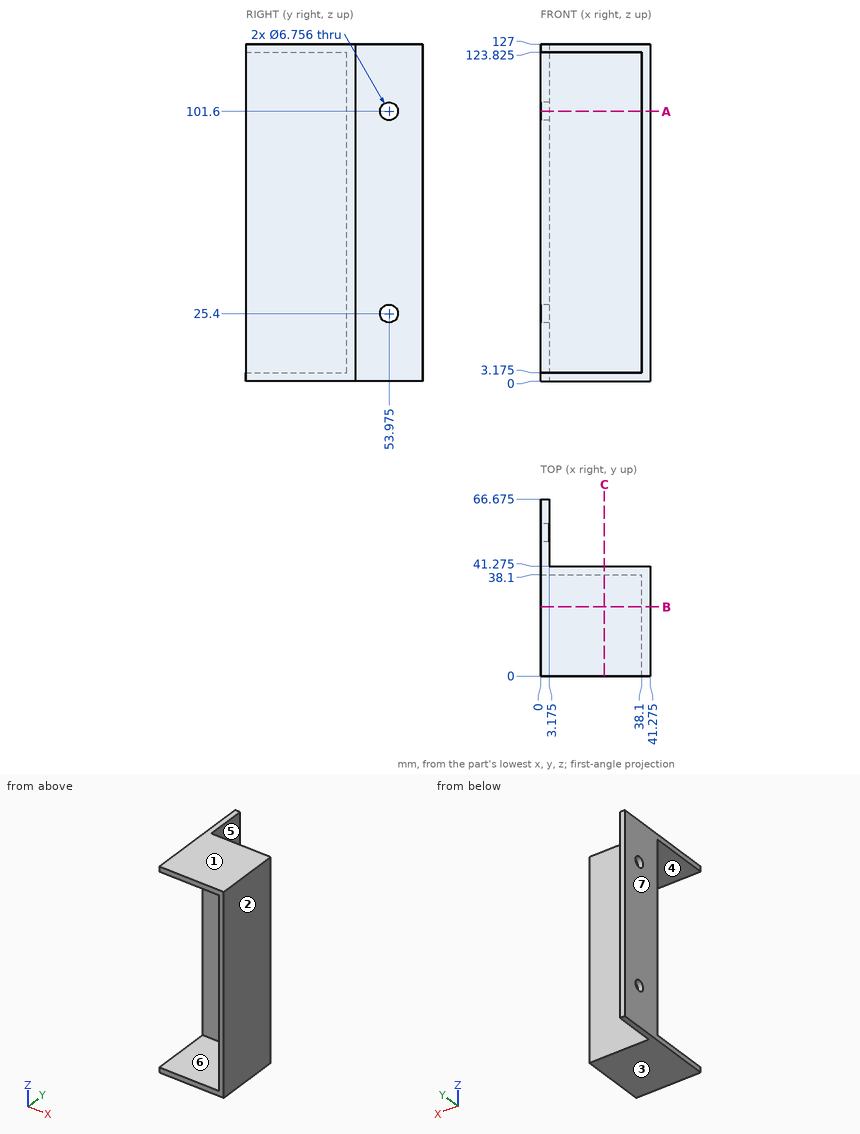
Source: three-view drawing plus pictorial views. Frame: mm from the lowest corner of the part. A direction names the side the tool comes from. Coordinates: 2 decimals unless noted, no trailing zeros. Order: outer loops, then holes, each group sorted by start corner. A loop starts at its lowest first (then second) coordinate and runs counter-clockwise, first axis right, second up.
Item 1: Set-up query: the marked faces 5, 6 and 7. Return all of +Z, -Z, +X, -X, +Y, -Y with unobstructed straight access to the full face (end or side cutting, diameter ignored); none if empty.
Output values:
face 5: +Z, -Z, +X, +Y
face 6: -X, -Y
face 7: +Z, -Z, -X, +Y, -Y
Item 2: Cut plane A-A (z = 101.6). Return loops of the section in (x, y) (1 decimal).
Output values:
outline: (0, 38.1) - (38.1, 38.1) - (38.1, 0) - (41.3, 0) - (41.3, 41.3) - (3.2, 41.3) - (3.2, 50.6) - (0, 50.6) - close; (0, 57.4) - (3.2, 57.4) - (3.2, 66.7) - (0, 66.7) - close
Item 3: Material intervals for line 1 (Y direction, x = 1.4, z = 101.6) (1 decimal); line 2 (Z direction, x = 4, y = 24) (1 decimal); line 3 (Y direction, x = 2, z = 25) (1 decimal), sorted ascending.
Output values:
line 1: y = 38.1 to 50.6, 57.4 to 66.7
line 2: z = 0 to 3.2, 123.8 to 127
line 3: y = 38.1 to 50.6, 57.3 to 66.7
Item 4: Cut plane B-B (y = 26). Return loops of the section in (x, z) (1 decimal).
Output values:
outline: (0, 0) - (41.3, 0) - (41.3, 127) - (0, 127) - (0, 123.8) - (38.1, 123.8) - (38.1, 3.2) - (0, 3.2) - close
Item 5: First-contact query: P1, Ø2, axis at x = 26, z = 36, coming from the +Y side (3 decimals); P2, Ø12.5, axis at y = 48, z = 41, coming from the +X side (3 decimals); P3, Ø1, axis at x = 23.5, z = 16.5, coming from the -Y side. Flat tips, straight axial feed; report the tip coordinate or a pass-through.
Output values:
P1: stops at y = 41.275
P2: stops at x = 3.175
P3: stops at y = 38.1
Item 6: Pull-direction query (Z, two-part tool) for the marked faces 1, 2, 3 and 4; classes: pulls with the +Z half, pulls with the -Z half, needs draft (parallel to the pull), parting line crosses it, or undercut.
Output values:
face 1: pulls with the +Z half
face 2: needs draft
face 3: pulls with the -Z half
face 4: undercut
